Source: CAD feature listing. Evaluate the final solid. Frame: model axes, mm. Face numbers are marked on the shaded views. A direction names the side the tool comes from. Give positions to 0.01 mm unless a question says otherwise; leave off trailing zeros. Order: outer loops, then holes, each group sorted by start corner. A loop starts at its lowest first (then second) coordinate and runs counter-clockwise, first axis right, second up.
1) Section C-C, the plane z = 14.5. Return loops of the section in (x, y), plus the area to 3 significant figures.
2) Section D-D, the plane x = 0.25. Give the number of separate pieces and of enclosed holes in the cut face, plus the area to 3 significant figures.
3) Material intervals for line 1 (Y direction, x = -0.5, z = 0); line 2 (Y direction, x = 5, z = 0); line 3 (Z direction, x = -3, y = -12.5), sorted ascending.
4) Access query for the marked faces 5, 6, 7 and 8. Directions: +Z, -Z, +X, -X, +Y, -Y. A direction counts if a zero-diameter tool reaches every point of the face in a straight line with its end or side. Return the directions, or none.
5) Draft query along Y for the marked faces 1, 2, 3 and 4. Return one class per face: released by +Y, released by -Y, zero draft, split by the parting line, or undercut.
6) Section B-B, the plane y = 0. Return loops of the section in (x, z).
7) Section A-A, the plane z = 0. Return loops of the section in (x, y), plus the area to 3 significant figures.
8) First-contact query: P1, Ø6, axis at x = -0.5, z = 14, coming from the -Y side; P2, Ø0.8, axis at x = 3.5, z = 20, coming from the +Y side; P3, Ø6, axis at x = -2.5, z = -18, coming from the +Y side. Flat tips, straight axial feed; report the tip coordinate or a pass-through.
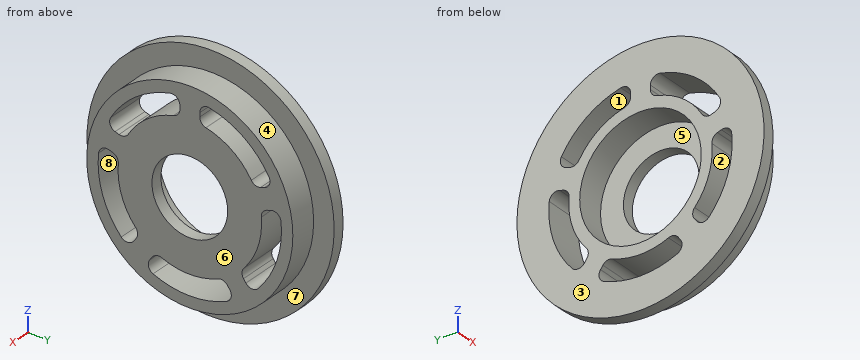
```python
from build123d import *

# Parameters (mm, degrees)
F3_DEPTH = 25


with BuildPart() as f1:
    # F0 (on Top) → F1 (revolve)
    with BuildSketch(Plane.XY):
        Polygon((-3.832785, 31), (-3.832785, 15.25), (3.167215, 15.25), (3.167215, 9.5), (6.167215, 9.5), (6.167215, 25.85), (-0.832785, 25.85), (-0.832785, 31), align=None)
    revolve(axis=Axis((4.667215, 0, 0), (-1, 0, 0)))

    # F2 (on face) → F3 (cut)
    with BuildSketch(Plane(origin=(-3.832785, 0, 0), x_dir=(0, -1, 0), z_dir=(-1, 0, 0))):
        with BuildLine():
            ThreePointArc((-2.5, 20.512191), (-3.246434, 22.070579), (-4.928571, 22.465734))
            ThreePointArc((-4.928571, 22.465734), (-13.519061, 18.607391), (-19.84317, 11.629643))
            ThreePointArc((-19.84317, 11.629643), (-19.987165, 9.907726), (-18.735711, 8.716257))
            Line((-18.735711, 8.716257), (-17.760863, 8.39951))
            ThreePointArc((-17.760863, 8.39951), (-16.442461, 8.428261), (-15.428546, 9.27146))
            ThreePointArc((-15.428546, 9.27146), (-10.580135, 14.562306), (-4.05, 17.538458))
            ThreePointArc((-4.05, 17.538458), (-2.934752, 18.242185), (-2.5, 19.487175))
            Line((-2.5, 19.487175), (-2.5, 20.512191))
        make_face()
        with BuildLine():
            ThreePointArc((4.928571, 22.465734), (3.246434, 22.070579), (2.5, 20.512191))
            Line((2.5, 20.512191), (2.5, 19.487175))
            ThreePointArc((2.5, 19.487175), (2.934752, 18.242185), (4.05, 17.538458))
            ThreePointArc((4.05, 17.538458), (10.580135, 14.562306), (15.428546, 9.27146))
            ThreePointArc((15.428546, 9.27146), (16.442461, 8.428261), (17.760863, 8.39951))
            Line((17.760863, 8.39951), (18.735711, 8.716257))
            ThreePointArc((18.735711, 8.716257), (19.987165, 9.907726), (19.84317, 11.629643))
            ThreePointArc((19.84317, 11.629643), (13.519061, 18.607391), (4.928571, 22.465734))
        make_face()
        with BuildLine():
            ThreePointArc((22.889195, 2.254943), (21.993571, 3.732642), (20.280796, 3.960974))
            Line((20.280796, 3.960974), (19.305948, 3.644227))
            ThreePointArc((19.305948, 3.644227), (18.256238, 2.84603), (17.931583, 1.567903))
            ThreePointArc((17.931583, 1.567903), (17.119017, -5.562306), (13.585366, -11.80838))
            ThreePointArc((13.585366, -11.80838), (13.096752, -13.033234), (13.476817, -14.295993))
            Line((13.476817, -14.295993), (14.079306, -15.125248))
            ThreePointArc((14.079306, -15.125248), (15.599181, -15.947268), (17.192325, -15.278219))
            ThreePointArc((17.192325, -15.278219), (21.8743, -7.107391), (22.889195, 2.254943))
        make_face()
        with BuildLine():
            ThreePointArc((9.217729, -21.072102), (10.346341, -19.763679), (10.034221, -18.064175))
            Line((10.034221, -18.064175), (9.431732, -17.234919))
            ThreePointArc((9.431732, -17.234919), (8.348223, -16.483242), (7.032328, -16.569441))
            ThreePointArc((7.032328, -16.569441), (0, -18), (-7.032328, -16.569441))
            ThreePointArc((-7.032328, -16.569441), (-8.348223, -16.483242), (-9.431732, -17.234919))
            Line((-9.431732, -17.234919), (-10.034221, -18.064175))
            ThreePointArc((-10.034221, -18.064175), (-10.346341, -19.763679), (-9.217729, -21.072102))
            ThreePointArc((-9.217729, -21.072102), (0, -23), (9.217729, -21.072102))
        make_face()
        with BuildLine():
            ThreePointArc((-17.192325, -15.278219), (-15.599181, -15.947268), (-14.079306, -15.125248))
            Line((-14.079306, -15.125248), (-13.476817, -14.295993))
            ThreePointArc((-13.476817, -14.295993), (-13.096752, -13.033234), (-13.585366, -11.80838))
            ThreePointArc((-13.585366, -11.80838), (-17.119017, -5.562306), (-17.931583, 1.567903))
            ThreePointArc((-17.931583, 1.567903), (-18.256238, 2.84603), (-19.305948, 3.644227))
            Line((-19.305948, 3.644227), (-20.280796, 3.960974))
            ThreePointArc((-20.280796, 3.960974), (-21.993571, 3.732642), (-22.889195, 2.254943))
            ThreePointArc((-22.889195, 2.254943), (-21.8743, -7.107391), (-17.192325, -15.278219))
        make_face()
    extrude(amount=-F3_DEPTH, mode=Mode.SUBTRACT)


solid = f1.part
```
From the geometry:
1. outline: (-3.83, -27.4) - (-0.83, -27.4) - (-0.83, -21.4) - (6.17, -21.4) - (6.17, -17.85) - (-3.83, -17.85) - close; (-3.83, -10.67) - (6.17, -10.67) - (6.17, 10.67) - (-3.83, 10.67) - (-3.83, 4.72) - (3.17, 4.72) - (3.17, -4.72) - (-3.83, -4.72) - close; (-3.83, 17.85) - (6.17, 17.85) - (6.17, 21.4) - (-0.83, 21.4) - (-0.83, 27.4) - (-3.83, 27.4) - close
1. area: 254 mm2
2. separate pieces: 1
2. enclosed holes: 6
2. area: 868 mm2
3. line 1: y = -25.85 to -23, -18 to -15.25, 15.25 to 18, 23 to 25.85
3. line 2: y = -25.85 to -23, -18 to -9.5, 9.5 to 18, 23 to 25.85
3. line 3: z = -28.37 to -8.74, 8.74 to 12.95, 19.31 to 28.37
4. face 5: -X
4. face 6: +Z, -Z, +X, +Y, -Y
4. face 7: +X
4. face 8: +X, -X
5. face 1: undercut
5. face 2: undercut
5. face 3: zero draft
5. face 4: split by the parting line
6. outline: (-3.83, -31) - (-0.83, -31) - (-0.83, -25.85) - (6.17, -25.85) - (6.17, -23) - (-3.83, -23) - close; (-3.83, -18) - (6.17, -18) - (6.17, -9.5) - (3.17, -9.5) - (3.17, -15.25) - (-3.83, -15.25) - close; (-3.83, 15.25) - (3.17, 15.25) - (3.17, 9.5) - (6.17, 9.5) - (6.17, 25.85) - (-0.83, 25.85) - (-0.83, 31) - (-3.83, 31) - close
7. outline: (-3.83, -31) - (-0.83, -31) - (-0.83, -25.85) - (6.17, -25.85) - (6.17, -23) - (-3.83, -23) - close; (-3.83, -18) - (6.17, -18) - (6.17, -9.5) - (3.17, -9.5) - (3.17, -15.25) - (-3.83, -15.25) - close; (-3.83, 15.25) - (3.17, 15.25) - (3.17, 9.5) - (6.17, 9.5) - (6.17, 18) - (-3.83, 18) - close; (-3.83, 23) - (6.17, 23) - (6.17, 25.85) - (-0.83, 25.85) - (-0.83, 31) - (-3.83, 31) - close
7. area: 177 mm2
8. P1: stops at y = -28.98
8. P2: stops at y = 16.85
8. P3: stops at y = 27.13
